Can you work these out from the model? Positions are in its coordinate system, mm. A direction names the side the tool comes from. Coordinates: 2 decimals unless noted, no trailing zeros. Loops run counter-clockwise (first coordinate to the right, second up) from the corner with the lowest first, then second, coordinate; pieces in that order, holes last. Notation, with made-up numbers: (85.5, 27) -> (90.5, 27) arc R36 ccw to (90.5, 64) -> close; hole circle Ø11 at (88.25, -40). An arc over 180 degrees is marked (long way). Put each result on its own line as item: value. Start each with the question number.
Item 1: If we section it at A-A on y = 0: Please give me the cut outline in (x, z), plus the area to 3 significant figures.
Item 2: Please list where these lines run through material, in increasing order: L1, parallel to Z at x = 3.25, y = -2.25; L2, parallel to Z at x = 0, y = -1.5; L3, parallel to X at y = 8.5, z = -21.5. Write a range as from..to.
Item 3: If we section it at D-D on z = -8: Please give me the cut outline in (x, y).
Item 4: Will these pins go through, and if not, where does the flat tip stop? P1, Ø10, axis at y = 0, z = -33.5, coming from the -X side; P2, Ø4, axis at x = 4, z = 0, coming from the -Y side; P3, Ø4, axis at x = -1, z = -4, coming from the +Y side.
Item 5: If we section it at C-C on y = -4: Please give me the cut outline in (x, z), plus the area to 3 significant figures.
Item 6: If we section it at B-B on z = -23: Please give me the cut outline in (x, y), plus the area to 3 significant figures.
Item 7: We'd pull the mould along Z, two halves only. Please class faces 6 (the cylindrical face through (2.965, -9.715, -45.699)), 7 (the cylindrical face through (2.97, 0.33, -20.52)), 8 (the flat face through (1, -4.5, -3)): pulls with the +Z half, pulls with the -Z half, needs draft (parallel to the pull), parting line crosses it, or undercut.
Item 8: For faces 1 (the flat face through (3, 7, -12)), 2 (the flat face through (3, -7, -12)), 3 (the flat face through (0.5, 0, -26)), 4 (the flat face through (3, 0, -46)), 5 (the cylindrical face through (-3.604, -0.063, 4.155)), which set-ups out of +Z, -Z, +X, -X, +Y, -Y let a thin tool reach every point of the face, with its end or its side?
```python
from build123d import *

# Parameters (mm, degrees)
F0_R     = 5.5
F1_DEPTH = 4.5
F3_DEPTH = 9
F4_W     = 20
F4_H     = 34
F5_DEPTH = 5
F7_D     = 2.5
F9_D     = 5
F10_R    = 1


with BuildPart() as f1:
    # F0 (on Front) → F1 (new body, symmetric)
    with BuildSketch(Plane.XZ):
        Circle(F0_R)
    extrude(amount=F1_DEPTH, both=True)

    # F2 (on face) → F3 (join, through all)
    with BuildSketch(Plane.XZ.offset(4.5)):
        with BuildLine():
            Line((5.5, -46), (5.5, 0))
            ThreePointArc((5.5, 0), (4.0620192023, -3.7080992435), (0.5, -5.4772255751))
            Line((0.5, -5.4772255751), (0.5, -46))
            Line((0.5, -46), (5.5, -46))
        make_face()
    extrude(amount=-F3_DEPTH)

    # F4 (on face) → F5 (join, through all)
    with BuildSketch(Plane.YZ.offset(5.5)):
        with Locations((0, -29)):
            Rectangle(F4_W, F4_H)
    extrude(amount=-F5_DEPTH)

    # F7 (through all)
    with Locations(Plane.XZ.offset(4.5)):
        with Locations((0, 0)):
            Hole(F7_D / 2)

    # F9 (through all)
    with Locations(Plane.YZ.offset(5.5)):
        with Locations((0, -23)):
            Hole(F9_D / 2)

    # F10
    f10_edges = [f1.edges().sort_by_distance(p)[0] for p in [
        (0.5, 0, -5.477226),
        (3, -4.5, -12),
        (3, 4.5, -12),
        (3, 10, -12),
        (3, -10, -12),
        (3, -10, -46),
        (3, 10, -46),
    ]]
    fillet(f10_edges, radius=F10_R)


solid = f1.part
```
Solutions:
1. outline: (-0.42, -5.48) arc R1 cw to (0.5, -6.48) -> (0.5, -20.5) -> (5.5, -20.5) -> (5.5, 0) arc R5.5 ccw (long way) to start; (0.5, -46) -> (5.5, -46) -> (5.5, -25.5) -> (0.5, -25.5) -> close; hole circle Ø2.5 at (0, 0)
1. area: 274 mm^2
2. L1: -46..-24.09, -21.91..4.44
2. L2: -5.61..-1.25, 1.25..5.5
2. L3: 0.5..5.5
3. outline: (0.5, -4.5) -> (5.5, -4.5) -> (5.5, 4.5) -> (0.5, 4.5) -> close
4. P1: x = 0.5
4. P2: y = -4.5
4. P3: y = 4.5
5. outline: (-0.42, -5.48) arc R1 cw to (0.5, -6.48) -> (0.5, -46) -> (5.5, -46) -> (5.5, 0) arc R5.5 ccw (long way) to start; hole circle Ø2.5 at (0, 0)
5. area: 299 mm^2
6. outline: (0.5, -10) -> (5.5, -10) -> (5.5, -2.5) -> (0.5, -2.5) -> close; (0.5, 2.5) -> (5.5, 2.5) -> (5.5, 10) -> (0.5, 10) -> close
6. area: 75.0 mm^2
7. face 6: pulls with the -Z half
7. face 7: undercut
7. face 8: needs draft
8. face 1: +Z, +X, -X, +Y
8. face 2: +Z, +X, -X, -Y
8. face 3: -Z, -X, +Y, -Y
8. face 4: -Z, +X, -X, +Y, -Y
8. face 5: +Y, -Y
